Check sheet for the drawn part. Datum: minimum x, y, z corner. Units: mm. Give positions to 0.01 mm unless a question says otherwise; leave off trailing zeros. Loops run counter-clockwise (first coordinate to the right, second up) from the corner with the lowest first, then second, coordinate; pieces in that order, holes last. Notation, with made-up numbers: (89.5, 78.25) - (129.5, 78.25) arc R19 ccw to (129.5, 113.25) - close; hole circle Ø3 at (49, 80.5). An arc over 180 degrees is marked (long way). One line per item, written item: value. Start each with the question number.
1. Gauge pin test, flat ends, axial feed: pin 1 (0.9 mm diameter, centred on y = 54.5, z = 2, fed in from -X); pin 2 (0.9 mm diameter, centred on x = 50.5, z = 2, fed in from -Y); pin 3 (0.9 mm diameter, centred on y = 2.5, z = 1, fed in from -X). Record the tip position at first contact, or that the pin passes through.
2. Sectioned sample at B-B (y = 18). Record the cut outline in (x, z), plus the area to 3 significant figures.
3. Sectioned sample at A-A (z = 1.6). Record the cut outline in (x, y), plus the area to 3 significant figures.
4. Sectioned sample at C-C (x = 8). Record the cut outline in (y, z), plus the area to 3 significant figures.
5. Scan lines: L1, parallel to X at y = 62, z = 2.05; L2, parallel to X at y = 3.5, z = 2.75; L3, parallel to Y at x = 59.5, z = 1.7. Record each from-to range of solid material in increasing order. Write a range as [from, to].
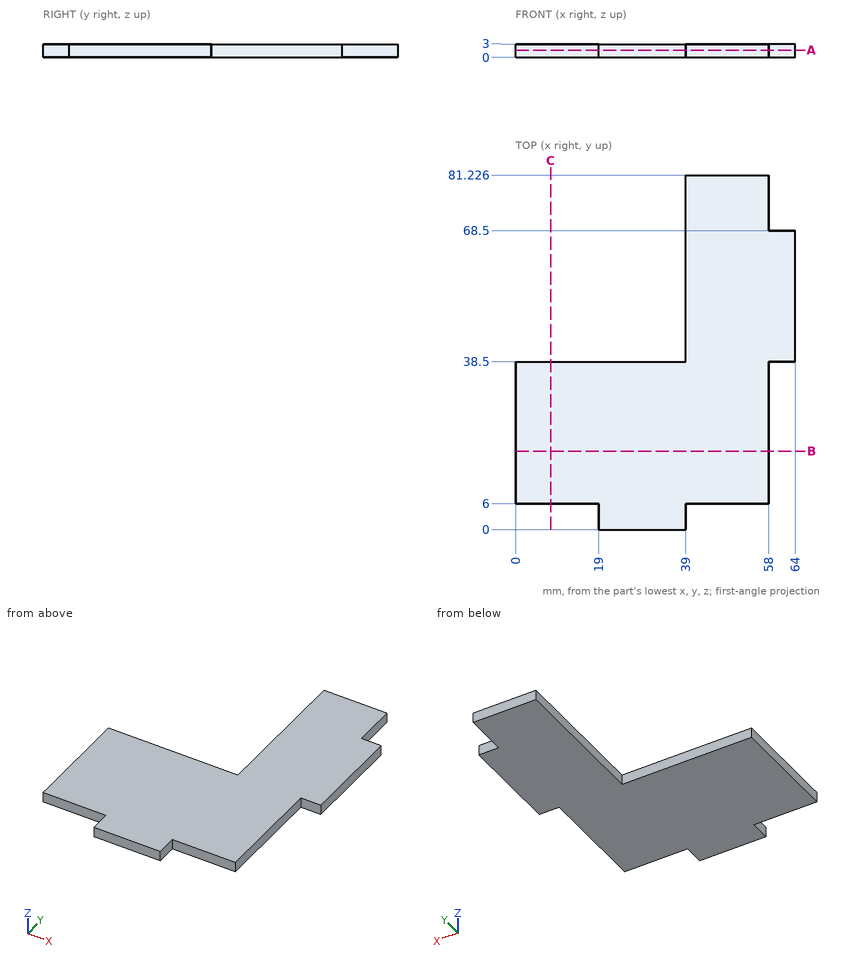
Results are:
1. pin 1: stops at x = 39
1. pin 2: stops at y = 6
1. pin 3: stops at x = 19
2. outline: (0, 0) - (58, 0) - (58, 3) - (0, 3) - close
2. area: 174 mm^2
3. outline: (0, 6) - (19, 6) - (19, 0) - (39, 0) - (39, 6) - (58, 6) - (58, 38.5) - (64, 38.5) - (64, 68.5) - (58, 68.5) - (58, 81.23) - (39, 81.23) - (39, 38.5) - (0, 38.5) - close
3. area: 3,000 mm^2
4. outline: (6, 0) - (38.5, 0) - (38.5, 3) - (6, 3) - close
4. area: 97.5 mm^2
5. L1: x = [39, 64]
5. L2: x = [19, 39]
5. L3: y = [38.5, 68.5]
